Read the model definition and answer for the solid it produces. Units are mm, in the model's axes. Face numbers are marked on the shaded views. Coordinates: 2 decimals unless noted, no trailing zeros. Order: outer loops, then holes, each group sorted by start corner. A loop starts at its lowest first (then second) coordinate and runs counter-clockwise, first axis right, second up.
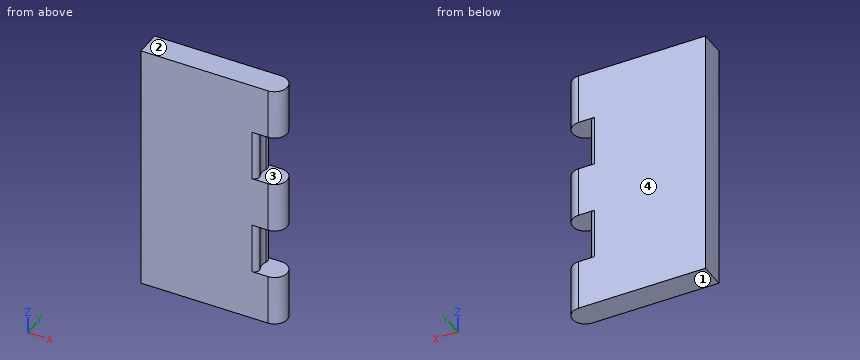
from build123d import *

# Parameters (mm, degrees)
SKETCH1_R      = 4.999999999999997
EXTRUDE1_DEPTH = 100
EXTRUDE3_START = 20
SKETCH1_5_R    = 4.999999999999997
EXTRUDE3_DEPTH = 20
EXTRUDE5_START = 60
SKETCH1_7_R    = 4.999999999999997
EXTRUDE5_DEPTH = 20
FILLET1_R      = 2


with BuildPart() as part:
    # Sketch1 → Extrude1 (new body)
    with BuildSketch(Plane.XY):
        with Locations((50, 5.000000000000032)):
            Circle(SKETCH1_R)
        Polygon((0, 0), (50, 2.082e-14), (50, 10.00000000000003), (-1.84e-15, 10.00000000000004), align=None)
    extrude(amount=EXTRUDE1_DEPTH)

    # Sketch1<5> → Extrude3 (cut)
    with BuildSketch(Plane.XY.offset(EXTRUDE3_START)):
        with Locations((50, 5.000000000000032)):
            Circle(SKETCH1_5_R)
    extrude(amount=EXTRUDE3_DEPTH, mode=Mode.SUBTRACT)

    # Sketch1<7> → Extrude5 (cut)
    with BuildSketch(Plane.XY.offset(EXTRUDE5_START)):
        with Locations((50, 5.000000000000032)):
            Circle(SKETCH1_7_R)
    extrude(amount=EXTRUDE5_DEPTH, mode=Mode.SUBTRACT)

    # Fillet1
    fillet1_edges = [part.edges().sort_by_distance(p)[0] for p in [
        (50, 10.00000000000003, 30),
        (50, 2.082e-14, 30),
        (50, 2.082e-14, 70),
        (50, 10.00000000000003, 70),
    ]]
    fillet(fillet1_edges, radius=FILLET1_R)


solid = part.part
Q1. The part is cut by section B-B, the plane z = 67.5. Determine the outline of the cut face in (x, y).
Q2. Straight lines are drawn through the part: L1, parallel to Z at x = 49, y = 6; L2, parallel to Y at x = 45.5, z = 79.5; L3, parallel to X at y = 7, z = 18.5. For each, find the intervals that lie inside material, in ascending order.
Q3. The part is cut by section A-A, the plane y = 5. Determine the outline of the cut face in (x, z).
Q4. Each of these flat-tipped pins is pushed along its axis until it touches: P1, Ø1, axis at y = 6, z = 76, coming from the +X side; P2, Ø1.5, axis at x = 38.5, y = 3, coming from the -Z side; P3, Ø4, axis at y = 1.5, z = 89.5, coming from the +X side. Where does it stop, or does it pass through?
Q5. Determine the mould class of the marked faces 1, 2, 3 and 4 for opening direction Z: +Z half, -Z half, draft (parallel to the pull), parting line (faces both ways), or undercut.
Q6. The part is cut by section C-C, the plane z = 14. Determine the outline of the cut face in (x, y).
Computed values:
1. outline: (0, 0) - (43.68, 0) arc R2 ccw to (45.48, 2.86) arc R5 cw to (45.48, 7.14) arc R2 ccw to (43.68, 10) - (0, 10) - close
2. L1: z = 0 to 20, 40 to 60, 80 to 100
2. L2: y = 1.18 to 2.82, 7.18 to 8.82
2. L3: x = 0 to 54.58
3. outline: (0, 0) - (55, 0) - (55, 20) - (45, 20) - (45, 40) - (55, 40) - (55, 60) - (45, 60) - (45, 80) - (55, 80) - (55, 100) - (0, 100) - close
4. P1: stops at x = 45.23
4. P2: stops at z = 0
4. P3: stops at x = 54.77
5. face 1: -Z half
5. face 2: +Z half
5. face 3: undercut
5. face 4: draft
6. outline: (0, 0) - (50, 0) arc R5 ccw to (50, 10) - (0, 10) - close
